Answer from the drawing. Dimensions are ordinates in mm from the lowest x, y and z of the part. A direction names the side the tool comes from. Coordinates: 2 decimals unless noted, no trailing zeros. Order: outer loops, then holes, each group sorted by start corner. A loop starts at its lowest first (then second) coordinate and runs counter-clockwise, first axis right, second up. Notation, with made-up numbers: M 54.5,80.25 L 75.5,80.25 A25 cw 75.5,113.25 Z; hole C 39.25,58.5 d2. An arc over 180 degrees is marked long. Use a Markdown table: item, result.
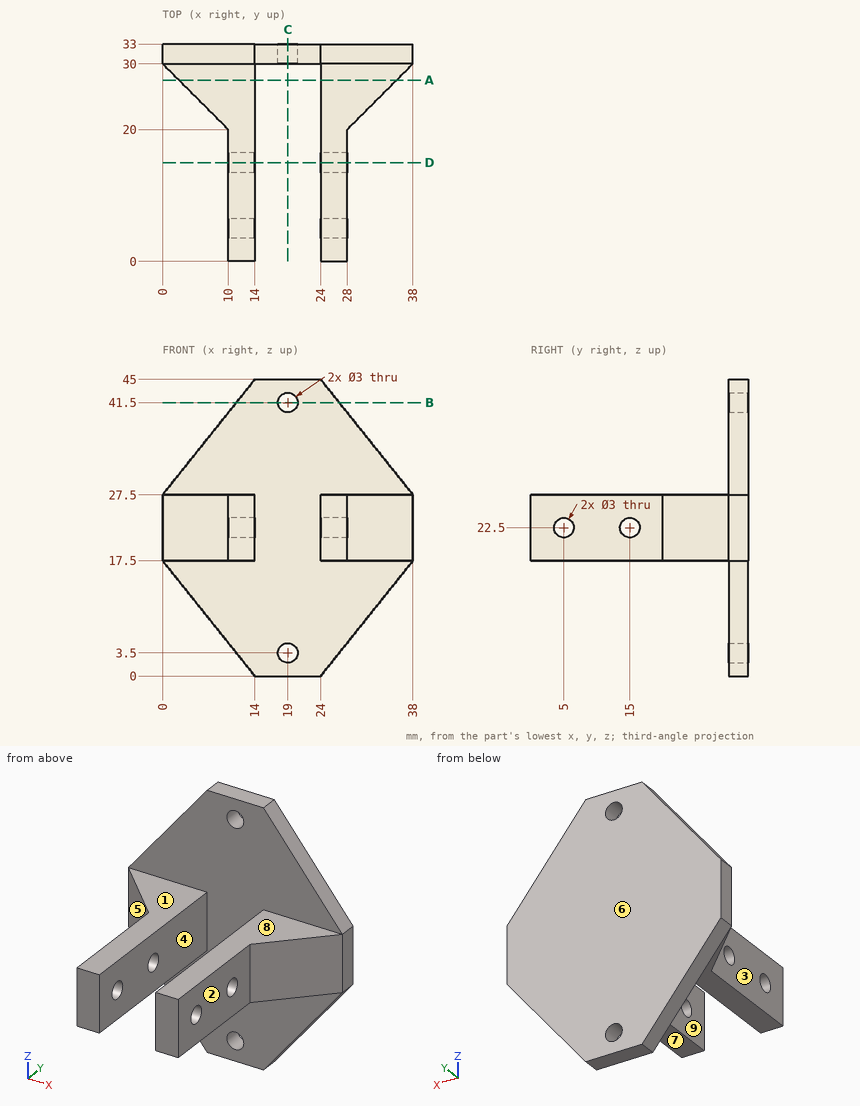
(1) A cutting plane is placed at A-A (y = 27.5). Determine the outline of the cut face in (x, z), then the cut area to 3 significant figures.
Conclusion:
| item | result |
|---|---|
| outline | M 2.5,17.5 L 14,17.5 L 14,27.5 L 2.5,27.5 Z; M 24,17.5 L 35.5,17.5 L 35.5,27.5 L 24,27.5 Z |
| area | 230 mm2 |
(2) A cutting plane is placed at D-D (y = 15). Determine the outline of the cut face in (x, z).
Conclusion:
| item | result |
|---|---|
| outline | M 10,17.5 L 14,17.5 L 14,21 L 10,21 Z; M 10,24 L 14,24 L 14,27.5 L 10,27.5 Z; M 24,17.5 L 28,17.5 L 28,21 L 24,21 Z; M 24,24 L 28,24 L 28,27.5 L 24,27.5 Z |
(3) A cutting plane is placed at B-B (z = 41.5). Determine the outline of the cut face in (x, y).
Conclusion:
| item | result |
|---|---|
| outline | M 11.2,30 L 17.5,30 L 17.5,33 L 11.2,33 Z; M 20.5,30 L 26.8,30 L 26.8,33 L 20.5,33 Z |
(4) Determine the mould class of the marked faces 1, 2, 3 and 4 for opening direction X: pulls with the +X half, pulls with the -X half, needs draft (parallel to the pull), parting line crosses it, or undercut.
Conclusion:
| item | result |
|---|---|
| face 1 | needs draft |
| face 2 | pulls with the +X half |
| face 3 | pulls with the -X half |
| face 4 | undercut |
(5) Which of the six approach directions +Z, -Z, +X, -X, +Y, -Y give full straight-line access (tool end or side, diameter ignored) to the marked faces 5, 6, 7, 8 and 9?
Conclusion:
| item | result |
|---|---|
| face 5 | +Z, -Z, -X, -Y |
| face 6 | +Z, -Z, +X, -X, +Y |
| face 7 | -Z, +X, -X, -Y |
| face 8 | +Z, +X, -X, -Y |
| face 9 | +Z, -Z, -Y |
(6) A cutting plane is placed at C-C (x = 19). Determine the outline of the cut face in (y, z), then the cut area to 3 significant figures.
Conclusion:
| item | result |
|---|---|
| outline | M 30,0 L 33,0 L 33,2 L 30,2 Z; M 30,5 L 33,5 L 33,40 L 30,40 Z; M 30,43 L 33,43 L 33,45 L 30,45 Z |
| area | 117 mm2 |
(7) Straight lines are drawn through the part: L1, parallel to Z at x = 19, y = 31; L2, parallel to X at y = 2.5, z = 24.5; L3, parallel to Y at x = 13, z = 22.5. For each, find the intervals that lie inside material, in ascending order.
Conclusion:
| item | result |
|---|---|
| L1 | 0 to 2, 5 to 40, 43 to 45 |
| L2 | 10 to 14, 24 to 28 |
| L3 | 0 to 3.5, 6.5 to 13.5, 16.5 to 33 |
(8) Given P1, Ø3.5, axis at y = 5, z = 22.5, coming from the +X side; P2, Ø1, axis at x = 12, z = 16.5, coming from the -Y side; P3, Ø10, axis at x = 25, y = 16.5, coming from the -Z side; P4, Ø4, axis at x = 19, z = 3.5, coming from the +Y side, each flat-ended and moving along its own axis, determine where each tip first touches the part or whether it passes through.
Conclusion:
| item | result |
|---|---|
| P1 | x = 28 |
| P2 | y = 30 |
| P3 | z = 17.5 |
| P4 | y = 33 |
